```python
from build123d import *

# Parameters (mm, degrees)
SKETCH_1_W          = 310
SKETCH_1_H          = 43
EXTRUDE_1_DEPTH     = 3
SKETCH_2_W          = 40
SKETCH_2_H          = 310
EXTRUDE_2_DEPTH     = 3
FILLET_1_R          = 2
FILLET_2_R          = 2
FILLET_3_R          = 1
SKETCH_3_R          = 2.05
CUT_EXTRUDE_1_DEPTH = 44


with BuildPart() as part:
    # 草图1 → 凸台-拉伸1 (new body)
    with BuildSketch(Plane(origin=(0, 0, 0), x_dir=(0, 0, -1), z_dir=(1, 0, 0))):
        with Locations((155, 21.5)):
            Rectangle(SKETCH_1_W, SKETCH_1_H)
    extrude(amount=EXTRUDE_1_DEPTH)

    # 草图2 → 凸台-拉伸2 (add)
    with BuildSketch(Plane(origin=(0, 0, 0), x_dir=(1, 0, 0), z_dir=(0, 1, 0))):
        with Locations((-20, 155)):
            Rectangle(SKETCH_2_W, SKETCH_2_H)
    extrude(amount=EXTRUDE_2_DEPTH)

    # 圆角1
    fillet_1_edges = [part.edges().sort_by_distance(p)[0] for p in [
        (3, 0, -155),
    ]]
    fillet(fillet_1_edges, radius=FILLET_1_R)

    # 圆角2
    fillet_2_edges = [part.edges().sort_by_distance(p)[0] for p in [
        (0, 3, -155),
    ]]
    fillet(fillet_2_edges, radius=FILLET_2_R)

    # 圆角3
    fillet_3_edges = [part.edges().sort_by_distance(p)[0] for p in [
        (-40, 1.5, -310),
        (-40, 1.5, 0),
        (1.5, 43, 0),
        (1.5, 43, -310),
    ]]
    fillet(fillet_3_edges, radius=FILLET_3_R)

    # 草图3 → 切除-拉伸1 (cut, through all)
    with BuildSketch(Plane(origin=(3, 0, 0), x_dir=(0, 0, -1), z_dir=(1, 0, 0))):
        with Locations((20, 37)):
            Circle(SKETCH_3_R)
        with Locations((20, 9)):
            Circle(SKETCH_3_R)
        with Locations((290, 9)):
            Circle(SKETCH_3_R)
        with Locations((290, 37)):
            Circle(SKETCH_3_R)
    extrude(amount=-CUT_EXTRUDE_1_DEPTH, mode=Mode.SUBTRACT)


solid = part.part
```
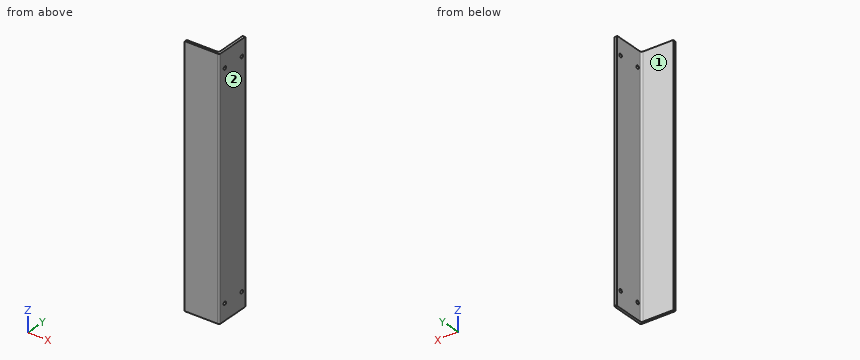
Check sheet for the modelled part. Datum: model origin and axes. Units: mm. Face numbers are marked on the shaded views. A direction names the side the tool comes from. Coordinates: 2 decimals unless noted, no trailing zeros. Loops run counter-clockwise (first coordinate to the right, second up) from the corner with the lowest first, then second, coordinate; pieces in that order, holes last.
1) Material ranges on probe 1 along Y at (x, z) = (1.5, -20); probe 2 along Y at (x, z) = (2, -20); probe 3 along X at (y, z) = (24, -95), recorded low to high.
2) Sectioned sample at A-A (z = -85). Record the boundary of the cut face in (x, y), and give its area (3 significant figures).
3) Sectioned sample at B-B (y = 28). Record the boundary of the cut face in (x, z).
4) Gauge pin test, flat ends, axial feed: pin 1 (4 mm diameter, centred on y = 13.5, z = -126, fed in from -X); pin 2 (12 mm diameter, centred on x = -25, z = -266, fed in from +Y); pin 3 (5 mm diameter, centred on y = 6, z = -278.5, fed in from -X). Record the tip position at first contact, or that the pin passes through.
5) Access from +Z, -Z, +X, -X, +Y, -Y to the whole of each face (thin tool, end or side, straight path). Record for the marked faces 1 and 2.
Check sheet entries:
1. probe 1: y = 0.06 to 6.95, 11.05 to 34.95, 39.05 to 43
1. probe 2: y = 0.27 to 6.95, 11.05 to 34.95, 39.05 to 43
1. probe 3: x = 0 to 3
2. outline: (-40, 0) - (1, 0) arc R2 ccw to (3, 2) - (3, 43) - (0, 43) - (0, 5) arc R2 cw to (-2, 3) - (-40, 3) - close
2. area: 249 mm2
3. outline: (0, -310) - (3, -310) - (3, 0) - (0, 0) - close
4. pin 1: stops at x = 0
4. pin 2: stops at y = 3
4. pin 3: stops at x = -0.68
5. face 1: +Z, -Z, -X, +Y
5. face 2: +Z, -Z, +X, +Y, -Y
